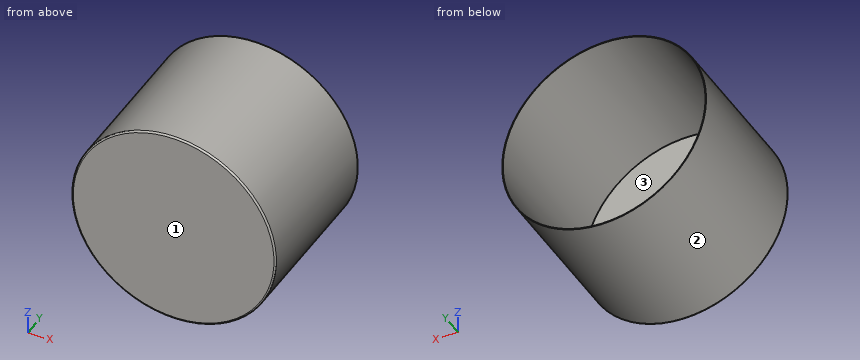
Autodesk Inventor part; units mm, degrees
ref_plane "YZ Plane" through (0, 0, 0) normal (1, 0, 0) x (0, 1, 0)
ref_plane "XZ Plane" through (0, 0, 0) normal (0, 1, 0) x (-1, 0, 0)
ref_plane "XY Plane" through (0, 0, 0) normal (0, 0, 1) x (1, 0, 0)
sketch "Sketch1" plane through (0, 0, 0) normal (0, 1, 0) x (-1, 0, 0)
  circle A0 centre (0, 0) radius 200
  dimension "d0" = 400
extrude "Extrusion1" add sketch "Sketch1" along normal blind 300
shell "Shell1" thickness 1 removed faces 1 at (26.6799, 300, 17.8469)
fillet "Fillet1" radius 3.175 1 edges at (200, 0, 0)
properties part number "distilate_tank"
Here's how the part is built. I have some questions about the finished solid (model axes, mm). Face numbers are marked on the shaded views. Round coordinates to 2 decimals unless told otherwise and drop trailing zeros. Order: outer loops, then holes, each group sorted by start corner. A loop starts at its lowest first (then second) coordinate and runs counter-clockwise, first axis right, second up. Notation, with made-up numbers: M 41.25,20 L 65.25,20 A16 ccw 65.25,34 Z; hole C 89,-2 d6. An arc over 180 degrees is marked long. Answer as CSV lines item,"result".
Item 1: Imagine slicing it at C-C on y = 266.5. List the corners of the cut face in (x, z) for me.
From the geometry:
outline,"C 0,0 d400; hole C 0,0 d398"
Item 2: Imagine slicing it at A-A on x = 0. List the corners of the cut face in (y, z) for me (3 decimals).
From the geometry:
outline,"M 0,-196.825 A3.175 ccw 3.175,-200 L 300,-200 L 300,-199 L 1,-199 L 1,199 L 300,199 L 300,200 L 3.175,200 A3.175 ccw 0,196.825 Z"
Item 3: Imagine slicing it at B-B on z = 0. List the corners of the cut face in (x, y) for me (3 decimals).
From the geometry:
outline,"M -200,3.175 A3.175 ccw -196.825,0 L 196.825,0 A3.175 ccw 200,3.175 L 200,300 L 199,300 L 199,1 L -199,1 L -199,300 L -200,300 Z"
Item 4: For pin 1 (10 mm diameter, centred on x = 31.5, z = -75.5, fed in from +Y); pin 2 (1 mm diameter, centred on y = 148, z = 69, fed in from +X); pin 3 (12 mm diameter, centred on y = 147, z = -38.5, fed in from -X), each with a flat end and sliding along its axis, tell me the tip position at first contact or that it passes through.
From the geometry:
pin 1,"y = 1"
pin 2,"x = 187.9"
pin 3,"x = -197.34"
Item 5: We'd pull the mould along X, two halves only. Please class the marked faces 1, 2 and 3: +X half, -X half, draft (parallel to the pull), parting line (faces both ways), or undercut.
From the geometry:
face 1,"draft"
face 2,"parting line"
face 3,"undercut"
Item 6: Please list where these lines run through material, in increasing order: L1, parallel to Z at x = 0, y = 214; L2, parallel to Y at x = 14, z = -143; L3, parallel to X at y = 22.5, z = 116. Write a range as [from, to].
From the geometry:
L1,"[-200, -199], [199, 200]"
L2,"[0, 1]"
L3,"[-162.92, -161.69], [161.69, 162.92]"
